from build123d import *

# Parameters (mm, degrees)
F0_R     = 85
F2_R     = 0.5
F4_R     = 105.9677495378
F5_DEPTH = 1


# Not quite as in the source:
# - a fillet or chamfer that OpenCascade refuses, or shapes differently, is made with other operations: its cross-section is extruded or revolved along the edge and cut away or added


with BuildPart() as f3:
    # F0 (on Top) → F3 section 0
    with BuildSketch(Plane.XY):
        Circle(F0_R)
    # F2 (on offset) → F3 section 1
    with BuildSketch(Plane.XY.offset(500)):
        Circle(F2_R)
    loft()

    # F4 (on Top) → F5 (join)
    with BuildSketch(Plane.XY):
        Circle(F4_R)
    extrude(amount=F5_DEPTH)

    # F6: fillet of radius 50 on 1 edges, made by hand

    # F6_s1 → F6_t2 (revolve)
    with BuildSketch(Plane.XZ):
        with BuildLine():
            ThreePointArc((105.9677495378, 1), (87.890537333, 15.9884437146), (78.6495736084, 37.5764875242))
            Line((78.6495736084, 37.5764875242), (84.831, 1))
            Line((84.831, 1), (105.9677495378, 1))
        make_face()
    revolve(axis=Axis((0, 0, 1), (0, 0, 1)))


solid = f3.part
The listing builds one solid part. Answer for the finished solid, in the listing's coordinates (mm). Coordinates: 2 decimals unless noted, no trailing zeros. Order: outer loops, then holes, each group sorted by start corner. A loop starts at its lowest first (then second) coordinate and runs counter-clockwise, first axis right, second up. Notation, with made-up numbers: (78, 39.25) -> (87, 39.25) arc R27 ccw to (87, 61.25) -> close; hole circle Ø1 at (72, 50). An arc over 180 degrees is marked (long way). Answer in a Markdown table with one row per item. Add a question column.
Item 1: Find section A-A (z = 224.5). Write down the section's boundary in (x, y), then the cut area to 3 significant figures.
Item 2: Find section B-B (z = 280.5). Write down the section's boundary in (x, y), then the cut area to 3 significant figures.
Item 3: Find the intervals of material crossed by L1, parallel to X at y = 21.5, z = 297; L2, parallel to Z at x = -56.5, y = 79; L3, parallel to X at y = -18, z = 334.5, in increasing order. Write a range as from..to.
Item 4: Each of these flat-tipped pins is pushed along its axis until it touches: P1, Ø4, axis at y = 30, z = 272, coming from the -X side; P2, Ø2, axis at x = 70, y = 52, coming from the +Z side; P3, Ø10, axis at x = 79.5, y = -70.5, coming from the -Z side; P4, Ø10, axis at x = 15, z = 65, coming from the +Y side. Where does it stop, or does it pass through?
Result set:
| question | item | result |
|---|---|---|
| 1 | outline | circle Ø94.12 at (0, 0) |
| 1 | area | 6,960 mm² |
| 2 | outline | circle Ø75.19 at (0, 0) |
| 2 | area | 4,440 mm² |
| 3 | L1 | x = -27.37..27.37 |
| 3 | L2 | z = 0..6.54 |
| 3 | L3 | x = -22.06..22.06 |
| 4 | P1 | stops at x = -27.25 |
| 4 | P2 | stops at z = 18.4 |
| 4 | P3 | stops at z = 0 |
| 4 | P4 | stops at y = 73.73 |
